from build123d import *

# Parameters (mm, degrees)
F0_W     = 70
F0_H     = 60
F0_W_2   = 50.823688
F0_H_2   = 36.305584
F1_DEPTH = 6
F2_W     = 70
F2_H     = 60
F2_W_2   = 60
F2_H_2   = 50
F3_DEPTH = 45
F5_D     = 5


with BuildPart() as f1:
    # F0 (on Top) → F1 (new body)
    with BuildSketch(Plane.XY):
        Rectangle(F0_W, F0_H)
        Rectangle(F0_W_2, F0_H_2, mode=Mode.SUBTRACT)
    extrude(amount=F1_DEPTH)

    # F2 (on face) → F3 (join)
    with BuildSketch(Plane(origin=(0, 0, 0), x_dir=(1, 0, 0), z_dir=(0, 0, -1))):
        Rectangle(F2_W, F2_H)
        Rectangle(F2_W_2, F2_H_2, mode=Mode.SUBTRACT)
    extrude(amount=F3_DEPTH)

    # F5 (through all)
    with Locations(Plane(origin=(0, 30, 0), x_dir=(-1, 0, 0), z_dir=(0, 1, 0))):
        with Locations((20, -40), (-11, -40), (4.5, -24.5), (20, -9), (-11, -9)):
            Hole(F5_D / 2)


solid = f1.part
Check sheet for the modelled part. Datum: model origin and axes. Units: mm. A direction names the side the tool comes from. Round coordinates to 2 decimals unless told otherwise and drop trailing zeros. Order: outer loops, then holes, each group sorted by start corner. A loop starts at its lowest first (then second) coordinate and runs counter-clockwise, first axis right, second up.
Q1. Cross-section at B-B, the plane x = -4.5. Enter the section's corners in (y, z), plus the area to 3 significant figures.
Filled sheet:
outline: (-30, -45) - (-25, -45) - (-25, -27) - (-30, -27) - close; (-30, -22) - (-25, -22) - (-25, 0) - (-18.15, 0) - (-18.15, 6) - (-30, 6) - close; (18.15, 0) - (25, 0) - (25, -22) - (30, -22) - (30, 6) - (18.15, 6) - close; (25, -45) - (30, -45) - (30, -27) - (25, -27) - close
area: 542 mm2
Q2. Depth check by flat-ended pin: P1, Ø6, axis at x = 11, z = -40, coming from the -Y side. Enter the tip coordinate at first touch or a pass-through.
Filled sheet:
P1: stops at y = -30
Q3. Cross-section at D-D, the plane x = 3. Enter the section's corners in (y, z).
Filled sheet:
outline: (-30, -45) - (-25, -45) - (-25, 0) - (-18.15, 0) - (-18.15, 6) - (-30, 6) - close; (18.15, 0) - (25, 0) - (25, -45) - (30, -45) - (30, 6) - (18.15, 6) - close
Q4. Set-up check for faces 1 (the face through (-22, -27.5, -10.5)), 2 (the face through (0, -25, -22)), 3 (the face through (0, 18.153, 3)): record each of +Z, -Z, +X, -X, +Y, -Y from which the full face is reachable in a straight line by a thin tool's end or side.
Filled sheet:
face 1: +Y, -Y
face 2: -Z
face 3: +Z, -Z
Q5. Draft check along Z on faces 4 (the face through (0, 20, 6)), 5 (the face through (-22.5, -27.5, -39.9)), 6 (the face through (30, 0, -22)). Enter one of: pulls with the +Z half, pulls with the -Z half, needs draft (parallel to the pull), parting line crosses it, or undercut.
Filled sheet:
face 4: pulls with the +Z half
face 5: undercut
face 6: needs draft
Q6. Cross-section at C-C, the plane z = -9. Enter the section's corners in (x, y), plus the area to 3 significant figures.
Filled sheet:
outline: (-35, -30) - (-22.5, -30) - (-22.5, -25) - (-30, -25) - (-30, 25) - (-22.5, 25) - (-22.5, 30) - (-35, 30) - close; (-17.5, -30) - (8.5, -30) - (8.5, -25) - (-17.5, -25) - close; (-17.5, 25) - (8.5, 25) - (8.5, 30) - (-17.5, 30) - close; (13.5, -30) - (35, -30) - (35, 30) - (13.5, 30) - (13.5, 25) - (30, 25) - (30, -25) - (13.5, -25) - close
area: 1,100 mm2
Q7. Cross-section at A-A, the plane y = 2.5. Enter the section's corners in (x, z).
Filled sheet:
outline: (-35, -45) - (-30, -45) - (-30, 0) - (-25.41, 0) - (-25.41, 6) - (-35, 6) - close; (25.41, 0) - (30, 0) - (30, -45) - (35, -45) - (35, 6) - (25.41, 6) - close
Q8. Scan lines: L1, parallel to Z at x = -20, y = -26; L2, parallel to X at y = -4, z = -6; L3, parallel to Y at x = 3, z = 3.5. Record each from-to range of solid material in increasing order.
Filled sheet:
L1: z = -45 to -42.5, -37.5 to -11.5, -6.5 to 6
L2: x = -35 to -30, 30 to 35
L3: y = -30 to -18.15, 18.15 to 30
